```python
from build123d import *

# Parameters (mm, degrees)
F1_W     = 126
F1_H     = 49
F1_W_2   = 120
F1_H_2   = 41
F2_DEPTH = 3
F3_DEPTH = 28.5
F5_DEPTH = 123
F6_R     = 2.5


with BuildPart() as f2:
    # F1 (on Top) → F2 (new body)
    with BuildSketch(Plane.XY):
        with Locations((0.1302100548, -8.2819438625)):
            Rectangle(F1_W, F1_H)
        with Locations((0.1302100548, -8.2819438625)):
            Rectangle(F1_W_2, F1_H_2, mode=Mode.SUBTRACT)
        with Locations((0.1302100548, -8.2819438625)):
            Rectangle(F1_W_2, F1_H_2)
    extrude(amount=-F2_DEPTH)

    # F1 (on Top) → F3 (join)
    with BuildSketch(Plane.XY):
        with Locations((0.1302100548, -8.2819438625)):
            Rectangle(F1_W, F1_H)
        with Locations((0.1302100548, -8.2819438625)):
            Rectangle(F1_W_2, F1_H_2, mode=Mode.SUBTRACT)
    extrude(amount=F3_DEPTH)

    # F4 (on face) → F5 (cut)
    with BuildSketch(Plane.YZ.offset(63.1302100548)):
        Polygon((12.2180561375, 28.5), (-28.7819438625, 28.5), (-29.9819438625, 24.5), (-28.7819438625, 24.5), (12.2180561375, 24.5), (13.4180561375, 24.5), align=None)
    extrude(amount=-F5_DEPTH, mode=Mode.SUBTRACT)

    # F6
    f6_edges = [f2.edges().sort_by_distance(p)[0] for p in [
        (63.13021, -32.781944, 12.75),
        (63.13021, 16.218056, 12.75),
        (-62.86979, -32.781944, 12.75),
        (-62.86979, 16.218056, 12.75),
        (0.13021, 16.218056, -3),
        (63.13021, -8.281944, -3),
        (0.13021, -32.781944, -3),
        (-62.86979, -8.281944, -3),
        (0.13021, -32.781944, 28.5),
        (-62.86979, -8.281944, 28.5),
        (0.13021, 16.218056, 28.5),
        (63.13021, 14.218056, 28.5),
        (63.13021, -30.781944, 28.5),
    ]]
    fillet(f6_edges, radius=F6_R)


solid = f2.part
```
The model under review builds one solid part; all positions refer to its coordinate system, in mm. A direction names the side the tool comes from. Round coordinates to 2 decimals unless told otherwise and drop trailing zeros. Order: outer loops, then holes, each group sorted by start corner. A loop starts at its lowest first (then second) coordinate and runs counter-clockwise, first axis right, second up. Notation, with made-up numbers: M 78,74 L 129,74 A26 cw 129,88 Z; hole C 60.5,41 d6. An arc over 180 degrees is marked long. Use a Markdown table: item, result.
1) Tool access review of faces 1 (the face through (60.13, -9, 12)), 2 (the face through (-62.87, -9, 13)): name each direction out of +Z, -Z, +X, -X, +Y, -Y from which nothing blocks a thin tool from reaching the whole face with its end or side.
Report:
| item | result |
|---|---|
| face 1 | +Z |
| face 2 | +Z, -Z, -X, +Y, -Y |
2) Consider section B-B (z = 17). Write out the cut boundary in (x, y).
Report:
| item | result |
|---|---|
| outline | M -62.87,-30.28 A2.5 ccw -60.37,-32.78 L 60.63,-32.78 A2.5 ccw 63.13,-30.28 L 63.13,13.72 A2.5 ccw 60.63,16.22 L -60.37,16.22 A2.5 ccw -62.87,13.72 Z; hole M -59.87,-28.78 L 60.13,-28.78 L 60.13,12.22 L -59.87,12.22 Z |
3) Draft analysis for pull direction X (two halves, no side actions). For faces 3 (the face through (2.491, -29.374, 26.528)), 4 (the face through (-1, 12.218, 12)), 5 (the face through (-62.157, -7.974, -2.248)), 6 (the face through (62.417, 13.145, 27.748)), state which applies: released by +X, released by -X, zero draft, split by the parting line, or undercut.
Report:
| item | result |
|---|---|
| face 3 | zero draft |
| face 4 | undercut |
| face 5 | released by -X |
| face 6 | released by +X |
4) Insertion check: pin 1 (3 mm diameter, centred on x = 13, y = -14, fed in from +Z); pin 2 (8 mm diameter, centred on x = 12.5, y = -25, fed in from +Z). Each pin has a flat end and moves straight along its axis. Give the tip position at first contact, or say it passes through.
Report:
| item | result |
|---|---|
| pin 1 | z = 0 |
| pin 2 | z = 28.5 |
5) Wall thickness on line 1 along X through (y, z) = (1, 7.5); line 2 along Y through (x, z) = (-38, 10); line 3 along Z through (x, y) = (24, -16.5): over which ranges is each line inside the solid? List them lowest first. Write a range as [from, to].
Report:
| item | result |
|---|---|
| line 1 | [-62.87, -59.87], [60.13, 63.13] |
| line 2 | [-32.78, -28.78], [12.22, 16.22] |
| line 3 | [-3, 0] |
6) Consider section C-C (y = 7). Write out the cut boundary in (x, z), then the cut area to 3 significant figures.
Report:
| item | result |
|---|---|
| outline | M -62.87,-0.5 A2.5 ccw -60.37,-3 L 60.63,-3 A2.5 ccw 63.13,-0.5 L 63.13,24.5 L 60.13,24.5 L 60.13,0 L -59.87,0 L -59.87,28.5 L -60.37,28.5 A2.5 ccw -62.87,26 Z |
| area | 533 mm^2 |
7) Consider section A-A (x = 14). Write out the cut boundary in (y, z), then the cut area to 3 significant figures.
Report:
| item | result |
|---|---|
| outline | M -32.78,-0.5 A2.5 ccw -30.28,-3 L 13.72,-3 A2.5 ccw 16.22,-0.5 L 16.22,26 A2.5 ccw 13.72,28.5 L 12.22,28.5 L 13.42,24.5 L 12.22,24.5 L 12.22,0 L -28.78,0 L -28.78,24.5 L -29.98,24.5 L -28.78,28.5 L -30.28,28.5 A2.5 ccw -32.78,26 Z |
| area | 365 mm^2 |
